Answer from the drawing. Dimensions are ordinates in mm from the lowest x, y and z of the part. Round coordinates to 2 decimals unless told otherwise and drop trailing zeros. Loops run counter-clockwise (first coordinate to the right, second up) from the corner with the lowest first, then second, coordinate; pieces in that order, holes last.
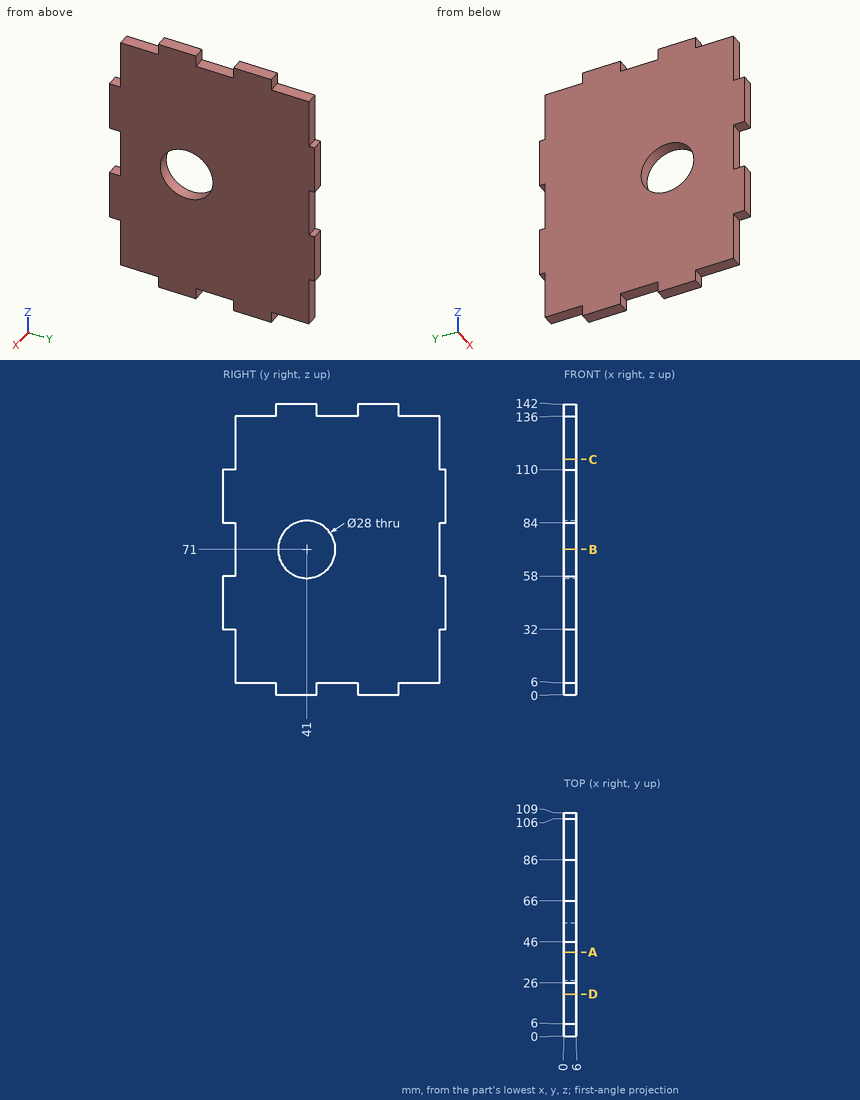
1. Consider probe 1 along Y at (x, z) = (1.75, 71); probe 2 along Y at (x, z) = (4.65, 10); probe 3 along Z at (x, y) = (4.3, 62.5). Determine where each line is inside the solid, lowest interval first.
Answer key:
probe 1: y = 6 to 27, 55 to 106
probe 2: y = 6 to 106
probe 3: z = 6 to 136
2. Find section C-C (z = 115). Write down the section's boundary in (x, y), then the cut area to 3 significant figures.
Answer key:
outline: (0, 6) - (6, 6) - (6, 106) - (0, 106) - close
area: 600 mm2
3. Find section D-D (y = 20.5). Write down the section's boundary in (x, z).
Answer key:
outline: (0, 6) - (6, 6) - (6, 136) - (0, 136) - close
4. Find section B-B (z = 71). Write down the section's boundary in (x, y).
Answer key:
outline: (0, 6) - (6, 6) - (6, 27) - (0, 27) - close; (0, 55) - (6, 55) - (6, 106) - (0, 106) - close
5. Find section A-A (y = 41). Write down the section's boundary in (x, z), then the cut area to 3 significant figures.
Answer key:
outline: (0, 0) - (6, 0) - (6, 57) - (0, 57) - close; (0, 85) - (6, 85) - (6, 142) - (0, 142) - close
area: 684 mm2
6. Given pin 1 (3 mm diameter, centred on x = 1.5, z = 2, fed in from +Y); pin 2 (1.5 mm diameter, centred on x = 2, y = 107.5, fed in from -Z); pin 3 (3.5 mm diameter, centred on x = 4, y = 108, fed in from +Z), each flat-ended and moving along its own axis, determine where each tip first touches the part or whether it passes through.
Answer key:
pin 1: stops at y = 86
pin 2: stops at z = 32
pin 3: stops at z = 110
